```python
from build123d import *

# Parameters (mm, degrees)
F1_W      = 60.5
F1_H      = 78.5
F2_DEPTH  = 21.5
F0_W      = 55.5
F0_H      = 73.5
F3_DEPTH  = 19.5
F4_W      = 78.5
F4_H      = 5
F5_DEPTH  = 2.5
F6_R      = 1.2
F7_DEPTH  = 25
F8_W      = 78.5
F8_H      = 5
F9_DEPTH  = 2.5
F10_R     = 1.2
F11_DEPTH = 25
F12_R     = 1.2
F13_DEPTH = 80
F14_W     = 44.0962035209
F14_H     = 7.4383728206
F15_DEPTH = 2.5


with BuildPart() as f2:
    # F1 (on Top) → F2 (new body)
    with BuildSketch(Plane.XY):
        with Locations((27.75, 36.75)):
            Rectangle(F1_W, F1_H)
    extrude(amount=F2_DEPTH)

    # F0 (on Top) → F3 (cut)
    with BuildSketch(Plane.XY):
        with Locations((27.75, 36.75)):
            Rectangle(F0_W, F0_H)
    extrude(amount=F3_DEPTH, mode=Mode.SUBTRACT)

    # F4 (on face) → F5 (join, through all)
    with BuildSketch(Plane.YZ.offset(58)):
        with Locations((36.75, -2.5)):
            Rectangle(F4_W, F4_H)
    extrude(amount=-F5_DEPTH)

    # F6 (on face) → F7 (cut)
    with BuildSketch(Plane.YZ.offset(58)):
        with Locations((1.5, 0.2)):
            Circle(F6_R)
        with Locations((6.5, 0.2)):
            Circle(F6_R)
    extrude(amount=-F7_DEPTH, mode=Mode.SUBTRACT)

    # F8 (on face) → F9 (join, through all)
    with BuildSketch(Plane(origin=(-2.5, 0, 0), x_dir=(0, -1, 0), z_dir=(-1, 0, 0))):
        with Locations((-36.75, -2.5)):
            Rectangle(F8_W, F8_H)
    extrude(amount=-F9_DEPTH)

    # F10 (on Right) → F11 (cut)
    with BuildSketch(Plane.YZ):
        with Locations((1.5, 0.2)):
            Circle(F10_R)
        with Locations((6.5, 0.2)):
            Circle(F10_R)
    extrude(amount=-F11_DEPTH, mode=Mode.SUBTRACT)

    # F12 (on face) → F13 (cut)
    with BuildSketch(Plane.XZ.offset(2.5)):
        with Locations((9.75, 8.75)):
            Circle(F12_R)
        with Locations((45.75, 8.75)):
            Circle(F12_R)
    extrude(amount=-F13_DEPTH, mode=Mode.SUBTRACT)

    # F14 (on face) → F15 (join, through all)
    with BuildSketch(Plane.XZ.offset(2.5)):
        with Locations((27.1060718223, 8.4709739313)):
            Rectangle(F14_W, F14_H)
    extrude(amount=-F15_DEPTH)


solid = f2.part
```
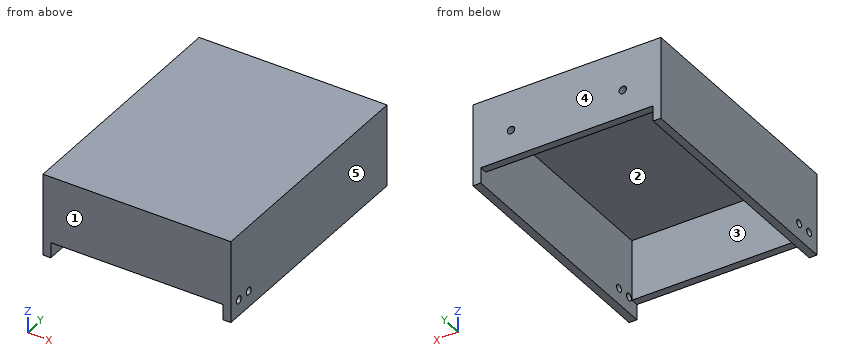
For this review, take the finished solid that the model builds, in its own axes (mm). Face numbers are marked on the shaded views. A direction names the side the tool comes from. Coordinates: 2 decimals unless noted, no trailing zeros. Write each loop counter-clockwise with the first axis right and the second up, starting at its lowest first coordinate (ties: lowest second). Pieces come first, ordered by that corner, then holes. Notation, with made-up numbers: (-32.75, 89.5) - (-13.75, 89.5) arc R18 cw to (-13.75, 112.5) - close; hole circle Ø8 at (14.25, -21.75). An arc over 180 degrees is marked (long way). Answer in a Markdown table with one row per item. Add a question column.
Q1. Draft analysis for pull direction X (two halves, no side actions). For the marked faces 3, 4 and 5, state which applies: +X half, -X half, draft (parallel to the pull), parting line (faces both ways), or undercut.
Q2. We need section C-C, the plane y = 6.5. State the section outline as (x, z) points, and give its area (4 significant figures).
Q3. For P1, Ø1.2, axis at x = 28, y = 74.5, coming from the -Z side; P2, Ø1.4, axis at y = 6.5, z = 0.2, coming from the +X side; P3, Ø1, axis at x = 12.5, y = 37.5, coming from the -Z side; P4, Ø4, axis at x = 9.75, z = 8.75, coming from the +Y side, all flat-tipped, find the tip position at first contact; note any pin that passes through.
Q4. For probe 1 along Y at (x, z) = (34, 1); probe 2 along X at (y, z) = (15, -2.25); probe 3 along Z at (x, y) = (57.1, 6.5), list the stretches that pass through material, from the lowest coordinate up.
Q5. We need section A-A, the plane x = 9.75. State the section outline as (y, z) points, and give its area (4 significant figures).
Q6. We need section D-D, the plane z = 3.5. State the section outline as (x, y) points.
Q7. Tool access review of the marked faces 1 and 2: name each direction out of +Z, -Z, +X, -X, +Y, -Y from which nothing blocks a thin tool from reaching the whole face with its end or side.
Q8. We need section B-B, the plane z = -3.5. State the section outline as (x, y) points, and give its area (4 significant figures).
Answer list:
| question | item | result |
|---|---|---|
| 1 | face 3 | undercut |
| 1 | face 4 | draft |
| 1 | face 5 | +X half |
| 2 | outline | (-2.5, -5) - (0, -5) - (0, -1) - (-2.5, -1) - close; (-2.5, 1.4) - (0, 1.4) - (0, 19.5) - (55.5, 19.5) - (55.5, 1.4) - (58, 1.4) - (58, 21.5) - (-2.5, 21.5) - close; (55.5, -5) - (58, -5) - (58, -1) - (55.5, -1) - close |
| 2 | area | 231.5 mm2 |
| 3 | P1 | stops at z = 0 |
| 3 | P2 | passes through |
| 3 | P3 | stops at z = 19.5 |
| 3 | P4 | stops at y = 76 |
| 4 | probe 1 | y = -2.5 to 0, 73.5 to 76 |
| 4 | probe 2 | x = -2.5 to 0, 55.5 to 58 |
| 4 | probe 3 | z = -5 to -1, 1.4 to 21.5 |
| 5 | outline | (-2.5, 0) - (0, 0) - (0, 19.5) - (73.5, 19.5) - (73.5, 9.95) - (76, 9.95) - (76, 21.5) - (-2.5, 21.5) - close; (73.5, 0) - (76, 0) - (76, 7.55) - (73.5, 7.55) - close |
| 5 | area | 248.5 mm2 |
| 6 | outline | (-2.5, -2.5) - (58, -2.5) - (58, 76) - (-2.5, 76) - close; hole (0, 0) - (55.5, 0) - (55.5, 73.5) - (0, 73.5) - close |
| 7 | face 1 | +Z, -Z, +X, -X, -Y |
| 7 | face 2 | -Z |
| 8 | outline | (-2.5, -2.5) - (0, -2.5) - (0, 76) - (-2.5, 76) - close; (55.5, -2.5) - (58, -2.5) - (58, 76) - (55.5, 76) - close |
| 8 | area | 392.5 mm2 |
